```python
from build123d import *

# Parameters (mm, degrees)
F0_W      = 188
F0_H      = 106
F1_DEPTH  = 5
F3_DEPTH  = 10
F4_R      = 2.877723
F4_R_2    = 3.098338
F4_R_3    = 3.080854
F4_R_4    = 2.682981
F5_DEPTH  = 25
F6_W      = 13.476193
F6_H      = 20.214289
F7_DEPTH  = 2
F6_H_2    = 37.733339
F6_W_2    = 15.834533
F6_H_3    = 12.128577
F6_W_3    = 21.561905
F6_H_4    = 13.139285
F8_DEPTH  = 6
F6_W_4    = 30.321434
F6_H_5    = 35.038095
F9_DEPTH  = 10
F10_W     = 11.828035
F10_H     = 15.372609
F10_W_2   = 7.715762
F10_H_2   = 12.800521
F11_DEPTH = 10
F12_W     = 9.468928
F12_H     = 12.915805
F13_DEPTH = 4
F14_W     = 3.46078
F14_H     = 10.265284
F15_DEPTH = 4


with BuildPart() as f1:
    # F0 (on Front) → F1 (new body)
    with BuildSketch(Plane.XZ):
        with Locations((-123.036315, 76.903633)):
            Rectangle(F0_W, F0_H)
    extrude(amount=F1_DEPTH)

    # F2 (on face) → F3 (join)
    with BuildSketch(Plane.XZ.offset(5)):
        Polygon((-47.522057, 127.648577), (-197.388828, 127.648577), (-214.953557, 110.367149), (-214.953557, 41.52476), (-198.23873, 26.226448), (-47.522057, 26.226448), (-31.373844, 41.52476), (-31.373844, 110.367149), align=None)
    extrude(amount=F3_DEPTH)

    # F4 (on face) → F5 (cut)
    with BuildSketch(Plane.XZ.offset(5)):
        with Locations((-211.029306, 123.802513)):
            Circle(F4_R)
        with Locations((-211.646155, 30.456685)):
            Circle(F4_R_2)
        with Locations((-36.373071, 30.164568)):
            Circle(F4_R_3)
        with Locations((-35.86828, 122.792944)):
            Circle(F4_R_4)
    extrude(amount=-F5_DEPTH, mode=Mode.SUBTRACT)

    # F6 (on face) → F7 (cut)
    with BuildSketch(Plane.XZ.offset(15)):
        with Locations((-177.695751, 76.344832)):
            Rectangle(F6_W, F6_H)
    extrude(amount=-F7_DEPTH, mode=Mode.SUBTRACT)

    # F6 (on face) → F8 (join)
    with BuildSketch(Plane.XZ.offset(15)):
        with Locations((-149.732649, 77.018644)):
            Rectangle(F6_W, F6_H_2)
        Polygon((-124.801703, 98.917454), (-131.876707, 98.917454), (-131.876707, 94.53769), (-131.876707, 86.788885), (-89.089796, 86.788885), (-89.089796, 98.917454), align=None)
        with Locations((-123.95944, 62.53174)):
            Rectangle(F6_W_2, F6_H_3)
        with Locations((-96.838608, 63.037093)):
            Rectangle(F6_W_3, F6_H_4)
    extrude(amount=F8_DEPTH)

    # F6 (on face) → F9 (join)
    with BuildSketch(Plane.XZ.offset(15)):
        with Locations((-63.148126, 74.323403)):
            Rectangle(F6_W_4, F6_H_5)
    extrude(amount=F9_DEPTH)

    # F10 (on face) → F11 (join)
    with BuildSketch(Plane.XZ.offset(25)):
        with Locations((-53.901426, 82.009707)):
            Rectangle(F10_W, F10_H)
        with Locations((-74.450962, 67.923142)):
            Rectangle(F10_W_2, F10_H_2)
    extrude(amount=F11_DEPTH)

    # F12 (on face) → F13 (cut)
    with BuildSketch(Plane.XZ.offset(35)):
        with Locations((-53.934842, 82.085251)):
            Rectangle(F12_W, F12_H)
    extrude(amount=-F13_DEPTH, mode=Mode.SUBTRACT)

    # F14 (on face) → F15 (cut)
    with BuildSketch(Plane.XZ.offset(35)):
        with Locations((-75.223997, 68.030607)):
            Rectangle(F14_W, F14_H)
    extrude(amount=-F15_DEPTH, mode=Mode.SUBTRACT)


solid = f1.part
```
For this review, take the finished solid that the model builds, in its own axes (mm). A direction names the side the tool comes from. Round coordinates to 2 decimals unless told otherwise and drop trailing zeros. Write each loop counter-clockwise with the first axis right and the second up, starting at its lowest first coordinate (ties: lowest second). Pieces come first, ordered by that corner, then holes. Notation, with made-up numbers: (30.25, -6) -> (37.25, -6) arc R20 cw to (37.25, 15) -> close; hole circle Ø9 at (-36.5, 27). An arc over 180 degrees is marked (long way). Use one line per item in the form item = value.
1) Take a section at C-C, the plane z = 51.5. Write out the cut boundary in (x, y), and give its area (3 significant figures).
Found:
outline = (-217.04, -5) -> (-214.95, -5) -> (-214.95, -15) -> (-31.37, -15) -> (-31.37, -5) -> (-29.04, -5) -> (-29.04, 0) -> (-217.04, 0) -> close
area = 2,780 mm2
2) To check wall thickness, follow L1, parallel to Z at x = -102.5, y = -20.5; L2, parallel to X at y = -17, z = 56.5; L3, parallel to Y at x = -154.5, z = 109. State the ranges of each line that lie inside material, in increasing order. Write a range as from..to.
Found:
L1 = 56.47..69.61, 86.79..98.92
L2 = -131.88..-116.04, -107.62..-86.06
L3 = -15..0
3) Tool access review of faces 1 (the flat face through (-54, -30, 74.323)), 2 (the flat face through (-97, -18, 69.607)), 3 (the flat face through (-59.815, -30, 82)): name each direction out of +Z, -Z, +X, -X, +Y, -Y from which nothing blocks a thin tool from reaching the whole face with its end or side.
Found:
face_1 = -Z, +X, -Y
face_2 = -Y
face_3 = +Z, -Z, -X, -Y
4) Take a section at B-B, the plane x = -180. Write out the cut boundary in (y, z), and give its area (3 significant figures).
Found:
outline = (-15, 26.23) -> (-5, 26.23) -> (-5, 23.9) -> (0, 23.9) -> (0, 129.9) -> (-5, 129.9) -> (-5, 127.65) -> (-15, 127.65) -> (-15, 86.45) -> (-13, 86.45) -> (-13, 66.24) -> (-15, 66.24) -> close
area = 1,500 mm2
5) Take a section at A-A, the plane y = -18. Write out the cut boundary in (x, z), and give its area (3 significant figures).
Found:
outline = (-156.47, 58.15) -> (-142.99, 58.15) -> (-142.99, 95.89) -> (-156.47, 95.89) -> close; (-131.88, 56.47) -> (-116.04, 56.47) -> (-116.04, 68.6) -> (-131.88, 68.6) -> close; (-131.88, 86.79) -> (-89.09, 86.79) -> (-89.09, 98.92) -> (-131.88, 98.92) -> close; (-107.62, 56.47) -> (-86.06, 56.47) -> (-86.06, 69.61) -> (-107.62, 69.61) -> close; (-78.31, 56.8) -> (-47.99, 56.8) -> (-47.99, 91.84) -> (-78.31, 91.84) -> close
area = 2,570 mm2
6) Take a section at D-D, the plane y = -8.5. Write out the cut boundary in (x, z).
Found:
outline = (-214.95, 41.52) -> (-198.24, 26.23) -> (-47.52, 26.23) -> (-31.37, 41.52) -> (-31.37, 110.37) -> (-47.52, 127.65) -> (-197.39, 127.65) -> (-214.95, 110.37) -> close
7) Clearance check with flat-ended pins moving along their axes: pin 1 (10 mm diameter, centred on x = -115, y = -21.5, fed in from -Z); pin 2 (3 mm diameter, centred on y = -32.5, z = 69.5, fed in from -X); pin 3 (11 mm diameter, centred on y = -30, z = 80.5, fed in from +X). State where each tip first meets the part, or that it passes through.
Found:
pin_1 = 56.47
pin_2 = -78.31
pin_3 = -47.99
8) Mouldability with a two-part tool opening along Z and no side actions: class faces 4 (the flat face through (-111, -21, 93)), 5 (the flat face through (-63, -20, 91.842)), 6 (the flat face through (-111, -18, 86.789)), 7 (the flat face through (-63, -20, 56.804)) as +Z half, -Z half, draft (parallel to the pull), parting line (faces both ways), or undercut.
Found:
face_4 = draft
face_5 = +Z half
face_6 = undercut
face_7 = -Z half
